Input: dimensioned drawing with shaded views. Units: mm. Origin: part minimum x, y, z. Round coordinates to 2 decimals unless told otherwise and drop trailing zeros. Loops run counter-clockwise (first coordinate to the right, second up) from the corner with the lowest first, then second, coordinate; pieces in that order, holes last. Notation, with made-up numbers: M 83,14.5 L 95,14.5 A21 cw 95,20.5 Z; hole C 11.5,-39 d1. An arc over 180 degrees is marked long. Use one line per item in the form item = value. Start each with the question number.
Q1. First-contact query: P1, Ø1.5, axis at x = 1, z = 5, coming from the +Y side; P2, Ø1.5, axis at y = 21, z = 3.5, coming from the +X side; P3, Ø8, axis at x = 40.5, y = 16.5, coming from the -Z side. Flat tips, straight axial feed; report the tip coordinate or a pass-through.
Q2. Ray query, line 1 along X through (y, z) = (11.5, 59); line 2 along Y through (x, z) = (19, 53); line 3 along Z through (x, y) = (36.5, 20.75). Return the intervals inside material, ascending.
Q3. Section query B-B, the plane z = 54. Output: boundary loops of the cut face in (x, y).
Q4. Mould query, pull axis X, two halves, no side actions, for the marked faces 1, 2, 3 and 4. Classes: pulls with the +X half, pulls with the -X half, needs draft (parallel to the pull), parting line crosses it, or undercut.
Q5. Section query D-D, the plane x = 24. Output: boundary loops of the cut face in (y, z), and give its area (3 significant figures).
Q6. Section query A-A, the plane y = 8. Output: boundary loops of the cut face in (x, z), and give its area (3 significant figures).
Q7. Section query C-C, the plane y = 16. Output: boundary loops of the cut face in (x, z).
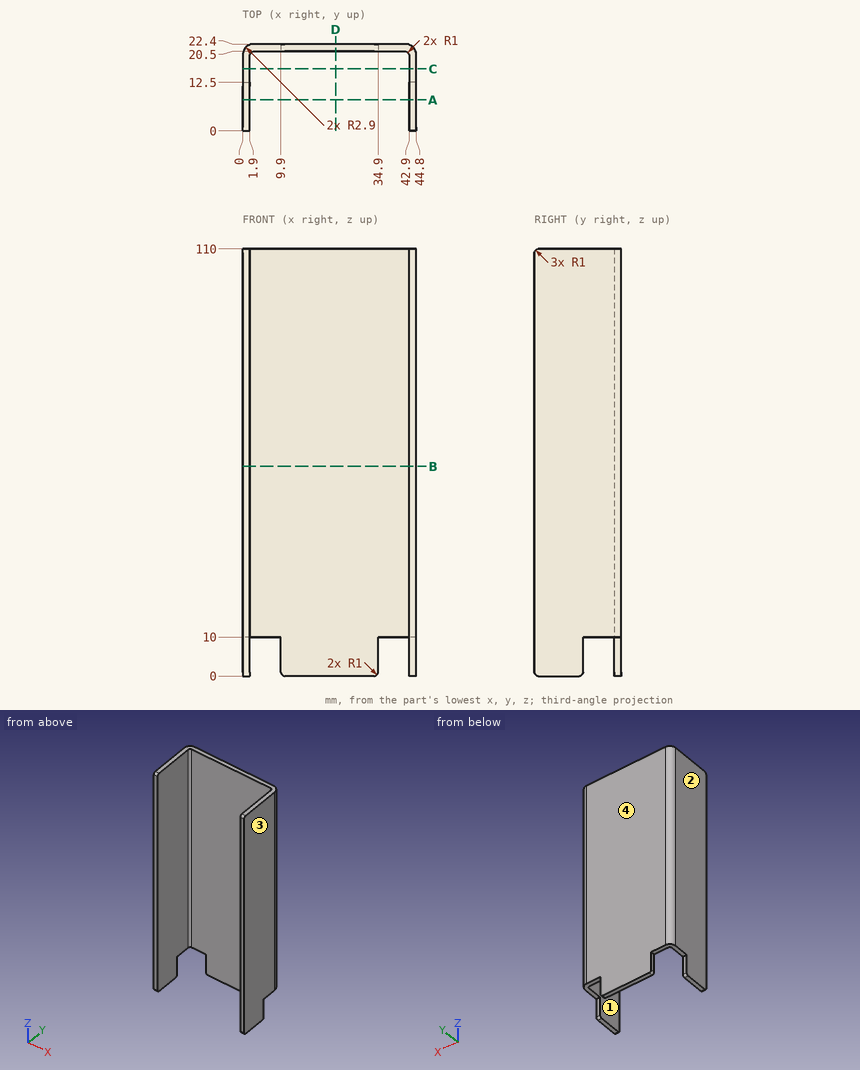
Results found:
q1.P1 = 12.5
q1.P2 = 34.9
q1.P3 = 10
q2.line_1 = 0 to 1.9, 42.9 to 44.8
q2.line_2 = 20.5 to 22.4
q2.line_3 = 10 to 110
q3.outline = M 0,0 L 1.9,0 L 1.9,19.5 A1 cw 2.9,20.5 L 41.9,20.5 A1 cw 42.9,19.5 L 42.9,0 L 44.8,0 L 44.8,19.5 A2.9 ccw 41.9,22.4 L 2.9,22.4 A2.9 ccw 0,19.5 Z
q4.face_1 = undercut
q4.face_2 = pulls with the -X half
q4.face_3 = pulls with the +X half
q4.face_4 = needs draft
q5.outline = M 20.5,0 L 22.4,0 L 22.4,110 L 20.5,110 Z
q5.area = 209 mm²
q6.outline = M 0,0 L 1.9,0 L 1.9,110 L 0,110 Z; M 42.9,0 L 44.8,0 L 44.8,110 L 42.9,110 Z
q6.area = 418 mm²
q7.outline = M 0,10 L 1.9,10 L 1.9,110 L 0,110 Z; M 42.9,10 L 44.8,10 L 44.8,110 L 42.9,110 Z
